The listing builds one solid part. Answer for the finished solid, in the listing's coordinates (mm). A direction names the side the tool comes from. Give positions to 0.01 mm unless a question says otherwise; leave off trailing zeros. Loops run counter-clockwise (first coordinate to the right, second up) from the corner with the lowest first, then second, coordinate; pieces in that order, holes last. Notation, with made-up numbers: (-14.75, 32) - (0.25, 32) arc R21 cw to (0.25, 48) - close; hole circle Ø11 at (-4, 12). An arc over 180 degrees is marked (long way). Write item = value, one per line. Start each with the question number.
1) Which of the six approach directions +Z, -Z, +X, -X, +Y, -Y give full straight-line access (tool end or side, diameter ignored) to faces 5 (the cylindrical face through (73.132, -5.993, 0.74)), 6 (the flat face through (73, -7, 1.5)), 7 (the flat face through (26, -13, 16)), 8 (the flat face through (74, -9, 10)), 9 (the flat face through (-1, -9, 22))?
2) The part is cut by section B-B on z = 12. Write down the section's boundary in (x, y).
3) Consider probe 1 along Z at (x, y) = (78, -4.75); probe 2 along Y at (x, z) = (26, 30); probe 3 along Z at (x, y) = (60, -10). Determine where each line is inside the solid, lowest interval first.
4) The part is cut by section A-A on x = 73. Write down the section's boundary in (y, z), plus the area to 3 significant figures.
5) Flat-ended cylindrical pins translate along their axes: P1, Ø4, axis at x = 26, y = -6, coming from the +Z side; P2, Ø3, axis at y = -12.5, z = 16, coming from the +X side; P3, Ø3, axis at x = 41.5, z = 15, coming from the +Y side; P4, Ø4.5, axis at y = -12.5, z = 19.5, coming from the -X side. Find the tip coordinate at first contact, or state that the pin passes through.
6) The part is cut by section C-C on y = -9.25. State how many separate pieces and enclosed holes the cut face has, plus the area to 3 significant figures.
7) The mould has two halves that part along X. Classify faces 1 (the flat face through (73, -7, 8.5)), 2 (the flat face through (-12, -7, 27)), 3 (the cylindrical face through (0, -6, 23)), 4 (the flat face through (84.7, 0, 4.9)): +X half, -X half, draft (parallel to the pull), parting line (faces both ways), or undercut.
8) The part is cut by section D-D on x = 0. Write down the section's boundary in (y, z), plus the area to 3 significant figures.
Autodesk Inventor part; units mm, degrees
ref_plane "РабПлоскость5" through (0, 0, 16) normal (0, 0, -1) x (-1, 0, 0)
ref_plane "РабПлоскость10" through (0, 0, 27) normal (0, 0, 1) x (1, 0, 0)
ref_plane "РабПлоскость11" through (0, 0, 5) normal (0, 0, -1) x (-1, 0, 0)
sketch "Эскиз1" plane through (0, 0, 0) normal (0, 0, 1) x (1, 0, 0)
  circle A0 centre (0, 0) radius 4
  circle A1 centre (0, 0) radius 11
  line L0 (-11, 0) -> (-12, 0)
  line L1 (-12, 0) -> (-12, -15)
  circle A2 centre (73, 0) radius 4
  circle A3 centre (73, 0) radius 11
  line L2 (84, 0) -> (85, 0)
  line L3 (85, 0) -> (85, -15)
  line L4 (-12, -15) -> (85, -15)
  line L5 (11, 0) -> (62, 0)
  dimension "d0" = 8
  dimension "d1" = 22
  dimension "d2" = 1
  dimension "d6" = 15
  dimension "d92" = 73
  dimension "d93" = 51
extrude "Выдавливание1" add sketch "Эскиз1" along normal blind 32 contours L5 A3 L2 L3 L4 L1 L0 A1
sketch "Эскиз2" plane through (0, 0, 32) normal (0, 0, 1) x (1, 0, 0)
  arc A0 (-11, 0) -> (11, 0) centre (0, 0) ccw
  line L0 (62, 0) -> (11, 0)
  arc A1 (-11, 0) -> (11, 0) centre (0, 0) ccw
  line L1 (11, 0) -> (11, 0)
  arc A2 (-6, 0) -> (6, 0) centre (0, 0) ccw
  line L2 (-11, 0) -> (-6, 0)
  line L3 (6, 0) -> (11, 0)
  dimension "d14" = 12
extrude "Выдавливание2" add sketch "Эскиз2" against normal blind 1.5
sketch "Эскиз3" plane through (0, 0, 32) normal (0, 0, 1) x (1, 0, 0)
  arc A0 (62, 0) -> (84, 0) centre (73, 0) ccw
  line L0 (85, 0) -> (84, 0)
  line L1 (84, 0) -> (84, 0)
  arc A1 (62, 0) -> (84, 0) centre (73, 0) ccw
  arc A2 (67.0053, 0) -> (78.9947, 0) centre (73, 0) ccw
  line L2 (62, 0) -> (11, 0)
  line L3 (62, 0) -> (67.0053, 0)
  line L4 (78.9947, 0) -> (84, 0)
  point P0 (0, 0)
extrude "Выдавливание3" add sketch "Эскиз3" against normal blind 1.5
ref_plane "РабПлоскость5" through (0, 0, 16) normal (0, 0, -1) x (-1, 0, 0)
mirror "Зеркальное отражение7" about plane through (0, 0, 16) normal (0, 0, -1) of "Выдавливание3"
mirror "Зеркальное отражение8" about plane through (0, 0, 16) normal (0, 0, -1) of "Выдавливание2"
ref_plane "РабПлоскость10" through (0, 0, 27) normal (0, 0, 1) x (1, 0, 0)
mirror "Зеркальное отражение9" about plane through (0, 0, 27) normal (0, 0, 1) of "Выдавливание2"
mirror "Зеркальное отражение10" about plane through (0, 0, 27) normal (0, 0, 1) of "Выдавливание3"
ref_plane "РабПлоскость11" through (0, 0, 5) normal (0, 0, -1) x (-1, 0, 0)
mirror "Зеркальное отражение11" about plane through (0, 0, 5) normal (0, 0, -1) of "Зеркальное отражение8"
mirror "Зеркальное отражение12" about plane through (0, 0, 5) normal (0, 0, -1) of "Зеркальное отражение7"
sketch "Эскиз14" plane through (6, 0, 30.5) normal (0, 1, 0) x (1, 0, 0)
  line L0 (5, 20.5) -> (5, 8.5)
  line L1 (5, 14.5) -> (56, 14.5)
  line L2 (56, 20.5) -> (56, 8.5)
  line L3 (56, 14.5) -> (56, 27)
  line L4 (56, 29) -> (56, 22)
  line L5 (5, 14.5) -> (5, 27)
  line L6 (5, 29) -> (5, 22)
  line L7 (5, 27) -> (56, 27)
  dimension "d94" = 12.5
extrude "Выдавливание11" cut sketch "Эскиз14" against normal blind 11
ref_plane "РабПлоскость14" through (36.5, -15, 0) normal (-1, 0, 0) x (0, 0, 1)
sketch "Эскиз15" plane through (85, 0, 32) normal (0, 1, 0) x (1, 0, 0)
  line L0 (-23, 16) -> (-23, 10)
  line L1 (-23, 10) -> (9, 10)
  line L2 (9, 10) -> (9, 22)
  line L3 (9, 22) -> (-23, 22)
  line L4 (-23, 22) -> (-23, 10)
  point P0 (-85, 32)
  dimension "d95" = 12
  dimension "d96" = 32
extrude "Выдавливание12" cut sketch "Эскиз15" against normal up to next
mirror "Зеркальное отражение15" about plane through (36.5, -15, 0) normal (-1, 0, 0) of "Выдавливание12"
sketch "Эскиз16" plane through (6, 0, 30.5) normal (0, 1, 0) x (1, 0, 0)
  line L0 (79, 8.5) -> (79, -1.5)
  line L1 (-18, 30.5) -> (-18, -1.5)
  line L2 (61.0053, -1.5) -> (0, -1.5)
  line L3 (30.5026, -1.5) -> (30.5026, 0.25)
  circle A0 centre (30.5026, 0.25) radius 1
  point P0 (-6, 30.5)
  point P1 (-18, 8.5)
  dimension "d86" = 1.75
  dimension "d87" = 2
extrude "Выдавливание13" cut sketch "Эскиз16" against normal up to next
mirror "Зеркальное отражение16" about plane through (0, 0, 16) normal (0, 0, -1) of "Выдавливание13"
mirror "Зеркальное отражение17" about plane through (0, 0, 16) normal (0, 0, -1) of "Выдавливание11"
sketch "Эскиз19" plane through (62, 0, 28.5) normal (0, 0, -1) x (-1, 0, 0)
  circle A0 centre (36, -6) radius 1.5
  line L0 (51, -11) -> (0, -11)
  line L1 (51, 0) -> (51, -11)
  point P0 (62, 0)
  dimension "d103" = 3
  dimension "d104" = 5
  dimension "d105" = 15
extrude "Выдавливание15" cut sketch "Эскиз19" against normal up to next
mirror "Зеркальное отражение18" about plane through (0, 0, 16) normal (0, 0, -1) of "Выдавливание15"
sketch "Эскиз20" plane through (6, -11, 30.5) normal (0, 1, 0) x (1, 0, 0)
  line L0 (5, 27) -> (56, 27)
  line L1 (5, 2) -> (56, 2)
  line L2 (5, 8.5) -> (5, 20.5)
  line L3 (5, 27) -> (56, 27)
  line L4 (56, 2) -> (5, 2)
  line L5 (15, 27) -> (20, 27)
  line L6 (20, 27) -> (20, 2)
  line L7 (20, 2) -> (15, 2)
  line L8 (15, 2) -> (15, 27)
  point P0 (-6, 30.5)
  dimension "d119" = 5
  dimension "d120" = 15
extrude "Выдавливание17" cut sketch "Эскиз20" against normal up to next
properties part number "Водило"
Answer below:
q1.face_5 = +Z, -Z, +Y
q1.face_6 = +Y
q1.face_7 = +Y, -Y
q1.face_8 = +X, +Y, -Y
q1.face_9 = -X, +Y, -Y
q2.outline = (11, -15) - (21, -15) - (21, -11) - (11, -11) - close; (26, -15) - (62, -15) - (62, -11) - (26, -11) - close
q3.probe_1 = 0 to 1.5, 8.5 to 10, 22 to 23.5, 30.5 to 32
q3.probe_2 = -15 to -7.5, -4.5 to 0
q3.probe_3 = 0 to 3.5, 28.5 to 32
q4.outline = (-15, 0) - (-5.99, 0) - (-5.99, 1.5) - (-11, 1.5) - (-11, 8.5) - (-5.99, 8.5) - (-5.99, 10) - (-15, 10) - close; (-15, 22) - (-5.99, 22) - (-5.99, 23.5) - (-11, 23.5) - (-11, 30.5) - (-5.99, 30.5) - (-5.99, 32) - (-15, 32) - close
q4.area = 110 mm2
q5.P1 = 32
q5.P2 = 62
q5.P3 = -11
q5.P4 = 11
q6.separate_pieces = 2
q6.enclosed_holes = 6
q6.area = 937 mm2
q7.face_1 = undercut
q7.face_2 = -X half
q7.face_3 = undercut
q7.face_4 = draft
q8.outline = (-15, 0) - (-6, 0) - (-6, 1.5) - (-11, 1.5) - (-11, 8.5) - (-6, 8.5) - (-6, 10) - (-15, 10) - close; (-15, 22) - (-6, 22) - (-6, 23.5) - (-11, 23.5) - (-11, 30.5) - (-6, 30.5) - (-6, 32) - (-15, 32) - close
q8.area = 110 mm2
